from build123d import *


with BuildPart() as f1:
    # F0 (on Front) → F1 (revolve)
    with BuildSketch(Plane.XZ):
        with BuildLine():
            Line((0, 0.5), (0, 0))
            Line((0, 0), (0, -7.5))
            Line((0, -7.5), (1, -7))
            Line((1, -7), (1, 0))
            Line((1, 0), (2.5, 0))
            Line((2.5, 0), (2.5, 0.5))
            Line((2.5, 0.5), (1.484474, 0.5))
            ThreePointArc((1.484474, 0.5), (1.277239, 1.00031), (0.776929, 1.207545))
            Line((0.776929, 1.207545), (0, 1.207545))
            Line((0, 1.207545), (0, 0.5))
        make_face()
    revolve(axis=Axis((0, 0, -3.75), (0, 0, -1)))


solid = f1.part
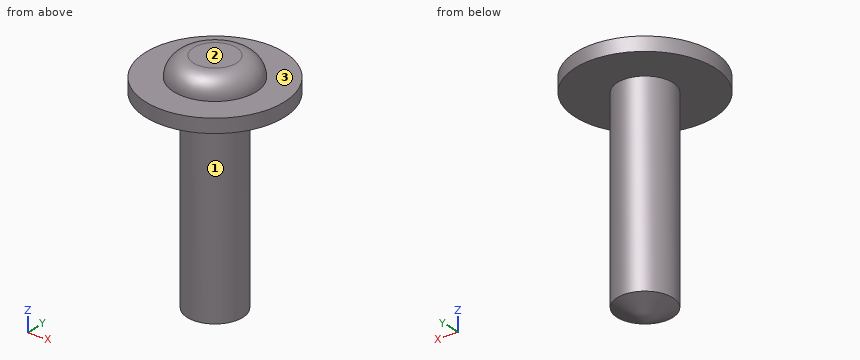
Geometry check sheet. Reference: the model listing, model coordinates, mm. Face numbers are marked on the shaded views. A direction names the side the tool comes from. Round coordinates to 2 decimals unless told otherwise and drop trailing zeros. Loops run counter-clockwise (first coordinate to the right, second up) from the corner with the lowest first, then second, coordinate; pieces in that order, holes last. Notation, with made-up numbers: (86, 36) -> (107, 36) arc R9 cw to (107, 42) -> close; hole circle Ø2 at (52.5, 81.5). An arc over 180 degrees is marked (long way). Answer as a JSON object with one key per item and string values. Group by question number.
Item 1: Cross-section at B-B, the plane x = 1.7. Record the cut outline in (y, z), plus the area to 3 significant figures.
Item 2: Set-up check for the marked faces 1, 2 and 3: record each of +Z, -Z, +X, -X, +Y, -Y from which the full face is reachable in a straight line by a thin tool's end or side.
Item 3: Thickness scan on line 1 along Z through (x, y) = (-1.65, 1.35); line 2 along X through (y, z) = (-0.05, -2.25); line 3 along Z through (x, y) = (-0.2, 0.05). Record the ranges inside material, lowest first.
Item 4: Cross-section at A-A, the plane z = -0.5. Record the cut outline in (x, y), plus the area to 3 significant figures.
Item 5: Cross-section at C-C, the plane y = -2.1. Record the cut outline in (x, z), plus the area to 3 significant figures.
Item 6: Depth check by flat-ended pin: pin 1 Ø1.5 at (x, y) = (1, 0) entering from -Z (3 decimals); pin 2 Ø3 at (x, z) = (0, -3) entering from -Y. Enter the tip coordinate at first touch or a pass-through.
Determined:
{
 "1": {"outline": "(-1.83, 0) -> (1.83, 0) -> (1.83, 0.5) -> (-1.83, 0.5) -> close", "area": "1.83 mm²"},
 "2": {"face 1": "-Z", "face 2": "+Z, +X, -X, +Y, -Y", "face 3": "+Z"},
 "3": {"line 1": "z = 0 to 0.5", "line 2": "x = -1 to 1", "line 3": "z = -7.4 to 1.21"},
 "4": {"outline": "circle Ø2 at (0, 0)", "area": "3.14 mm²"},
 "5": {"outline": "(-1.36, 0) -> (1.36, 0) -> (1.36, 0.5) -> (-1.36, 0.5) -> close", "area": "1.36 mm²"},
 "6": {"pin 1": "stops at z = -7.375", "pin 2": "stops at y = -1"}
}
